Geometry check sheet. Reference: the model listing, model coordinates, mm. A direction names the side the tool comes from. Coordinates: 2 decimals unless noted, no trailing zeros. Loops run counter-clockwise (first coordinate to the right, second up) from the corner with the lowest first, then second, coordinate; pieces in that order, holes last. Notation, with made-up numbers: (53.25, 51) - (74.25, 51) arc R21 ccw to (74.25, 57) - close; hole circle Ø11 at (67.5, 3.25). An arc over 180 degrees is marked (long way). One line per item, written item: value.
from build123d import *

# Parameters (mm, degrees)
ESBO_O1_R                = 20
RESSALTO_EXTRUS_O1_DEPTH = 2
ESBO_O2_R                = 5.1
RESSALTO_EXTRUS_O2_DEPTH = 5
ESBO_O3_R                = 1.55
CORTE_EXTRUS_O1_DEPTH    = 29.722813233
PADR_OCIRCULAR1_COUNT    = 4


with BuildPart() as part:
    # Esboço1 → Ressalto-extrusão1 (new body)
    with BuildSketch(Plane.XY):
        Circle(ESBO_O1_R)
    extrude(amount=RESSALTO_EXTRUS_O1_DEPTH)

    # Esboço2 → Ressalto-extrusão2 (add)
    with BuildSketch(Plane.XY.offset(2)):
        Circle(ESBO_O2_R)
    extrude(amount=RESSALTO_EXTRUS_O2_DEPTH)

    # Esboço3 → Corte-extrusão1 (cut, through all)
    with BuildSketch(Plane.XY.offset(2)):
        with Locations((12.5, 0)):
            Circle(ESBO_O3_R)
    corte_extrus_o1 = extrude(amount=-CORTE_EXTRUS_O1_DEPTH, mode=Mode.SUBTRACT)

    # PadrãoCircular1: Corte-extrusão1 ×4 about axis
    padr_ocircular1_axis = Axis((0, 0, 0), (0, 0, 1))
    for i in range(1, PADR_OCIRCULAR1_COUNT):
        add(corte_extrus_o1.rotate(padr_ocircular1_axis, i * 360 / PADR_OCIRCULAR1_COUNT), mode=Mode.SUBTRACT)


solid = part.part
(1) Cross-section at D-D on y = -12.5. Record the cut outline in (x, z).
Reply:
outline: (-15.61, 0) - (-1.55, 0) - (-1.55, 2) - (-15.61, 2) - close; (1.55, 0) - (15.61, 0) - (15.61, 2) - (1.55, 2) - close
(2) Access from +Z, -Z, +X, -X, +Y, -Y to the whole of each face (thin tool, end or side, straight path). Record for faces 1 (the face through (-11.27, 0.94, 1.01)), 2 (the face through (4, -4, 2)).
Reply:
face 1: +Z, -Z
face 2: +Z
(3) Go/stop test with flat-tipped pins: pin 1 Ø2.5 at (x, y) = (0, -12.5) entering from +Z; pin 2 Ø4 at (x, y) = (-0.5, 10) entering from +Z; pin 3 Ø1.5 at (y, z) = (3, 1) entering from -X; pin 4 Ø4 at (y, z) = (2.5, 3.5) entering from -X. Record where each tip stops, or that it passes through.
Reply:
pin 1: through
pin 2: z = 2
pin 3: x = -19.87
pin 4: x = -19.97
(4) Cross-section at C-C on z = 1. Record the cut outline in (x, y), and give its area (3 significant figures).
Reply:
outline: circle Ø40 at (0, 0); hole circle Ø3.1 at (-12.5, 0); hole circle Ø3.1 at (0, -12.5); hole circle Ø3.1 at (0, 12.5); hole circle Ø3.1 at (12.5, 0)
area: 1,230 mm2
(5) Cross-section at A-A on y = 0. Record the cut outline in (x, z), and give its area (3 significant figures).
Reply:
outline: (-20, 0) - (-14.05, 0) - (-14.05, 2) - (-20, 2) - close; (-10.95, 0) - (10.95, 0) - (10.95, 2) - (5.1, 2) - (5.1, 7) - (-5.1, 7) - (-5.1, 2) - (-10.95, 2) - close; (14.05, 0) - (20, 0) - (20, 2) - (14.05, 2) - close
area: 119 mm2
(6) Material ranges on probe 1 along Z at (x, y) = (-7, 4); probe 2 along X at (y, z) = (-12.5, 1.4), recorded low to high. Write a range as from..to.
Reply:
probe 1: 0..2
probe 2: -15.61..-1.55, 1.55..15.61
(7) Release check for a two-part mould opening along Y. For faces 3 (the face through (2.4, -4.5, 4.5)), 4 (the face through (0, 0, 0)), 5 (the face through (-0.94, -11.27, 1.01)) record: pulls with the +Y half, pulls with the -Y half, needs draft (parallel to the pull), parting line crosses it, or undercut.
Reply:
face 3: parting line crosses it
face 4: needs draft
face 5: undercut
